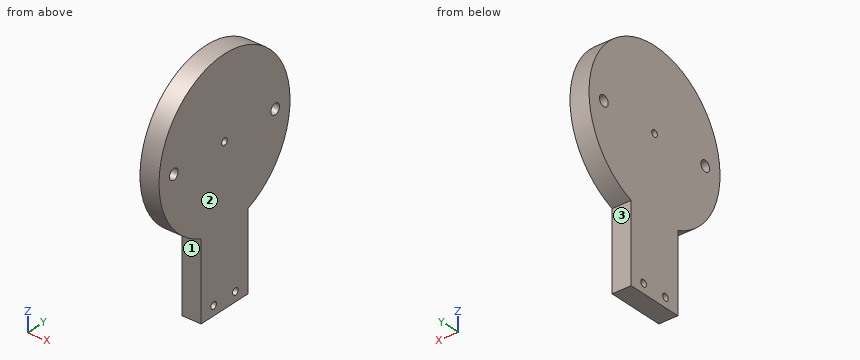
```python
from build123d import *

# Parameters (mm, degrees)
EXTRUDE_1_DEPTH     = 5
SKETCH_8_R          = 0.9
SKETCH_8_R_2        = 1.4
CUT_EXTRUDE_3_DEPTH = 10


with BuildPart() as part:
    # 스케치1 → 보스-돌출1 (new body)
    with BuildSketch(Plane(origin=(-9, 0, 0), x_dir=(0, -1, 0), z_dir=(-1, 0, 0))):
        with BuildLine():
            Line((-21, -18.122865071), (-21, 2.262089683))
            ThreePointArc((-21, 2.262089683), (-13.5, 42.877134929), (-6, 2.262089683))
            Line((-6, 2.262089683), (-6, -18.122865071))
            Line((-6, -18.122865071), (-21, -18.122865071))
        make_face()
    extrude(amount=-EXTRUDE_1_DEPTH)

    # 스케치8 → 컷-돌출3 (cut)
    with BuildSketch(Plane.ZY.offset(9)):
        with Locations((21.877134929, 13.5)):
            Circle(SKETCH_8_R)
        with Locations((-15.622865071, 17)):
            Circle(SKETCH_8_R)
        with Locations((-15.622865071, 10)):
            Circle(SKETCH_8_R)
        with Locations((21.877134929, 29.75)):
            Circle(SKETCH_8_R_2)
        with Locations((21.877134929, -2.75)):
            Circle(SKETCH_8_R_2)
    extrude(amount=-CUT_EXTRUDE_3_DEPTH, mode=Mode.SUBTRACT)


solid = part.part
```
Part model, mm, in its own coordinate system. Face numbers are marked on the shaded views. A direction names the side the tool comes from. Round coordinates to 2 decimals unless told otherwise and drop trailing zeros. Order: outer loops, then holes, each group sorted by start corner. A loop starts at its lowest first (then second) coordinate and runs counter-clockwise, first axis right, second up. Notation, with made-up numbers: M -27,15.5 L 29,15.5 A15 ccw 29,34.5 Z; hole C 6,-5 d10. An arc over 180 degrees is marked long. Answer in a Markdown table with one row per item. Add a question column.
Q1. Cut at B-B on x = -5.65. Give the cut face in (y, z), and give its area (3 significant figures).
Q2. Wall check: L1, parallel to Y at x = -7, z = -2; L2, parallel to Z at x = -7.45, y = 31; L3, parallel to Z at x = -6.6, y = 8. Give the ranges that are in metal, low to high. Write a range as from..to.
Q3. Cut at A-A on y = 30.5. Give the cut face in (x, z), and give its area (3 significant figures).
Q4. Pin check, flat tips, straight feed: pin 1 (1 mm diameter, centred on x = -5.5, y = 20, fed in from +Z); pin 2 (3 mm diameter, centred on x = -6.5, y = 8, fed in from +Z); pin 3 (1.1 mm diameter, centred on y = 17, z = -15.62, fed in from +X); pin 4 (3 mm diameter, centred on x = -7, z = 12.5, fed in from +Y). Stop position of each tip, or through.
Q5. Cut at C-C on z = -14. Give the cut face in (x, y), and give its area (3 significant figures).
Q6. 3-axis set-ups, long thin cutter, end or side, ignore diameter. For the marked faces 1, 2 and 3: which of +Z, -Z, +X, -X, +Y, -Y reach the whole face in a straight line?
Q7. Cut at D-D on y = 17. Give the cut face in (x, z), and give its area (3 significant figures).
Established:
| question | item | result |
|---|---|---|
| 1 | outline | M 6,-18.12 L 21,-18.12 L 21,2.26 A21 ccw long 6,2.26 Z; hole C -2.75,21.88 d2.8; hole C 10,-15.62 d1.8; hole C 13.5,21.88 d1.8; hole C 17,-15.62 d1.8; hole C 29.75,21.88 d2.8 |
| 1 | area | 1,660 mm2 |
| 2 | L1 | y = 6..21 |
| 2 | L2 | z = 10.27..21.25, 22.51..33.49 |
| 2 | L3 | z = -18.12..42.14 |
| 3 | outline | M -9,9.55 L -4,9.55 L -4,20.69 L -9,20.69 Z; M -9,23.06 L -4,23.06 L -4,34.21 L -9,34.21 Z |
| 3 | area | 111 mm2 |
| 4 | pin 1 | stops at z = 42 |
| 4 | pin 2 | stops at z = 42.49 |
| 4 | pin 3 | passes through |
| 4 | pin 4 | stops at y = 32.97 |
| 5 | outline | M -9,6 L -4,6 L -4,21 L -9,21 Z |
| 5 | area | 75.0 mm2 |
| 6 | face 1 | -Z, +X, -X, -Y |
| 6 | face 2 | +Z, -Z, +X, +Y, -Y |
| 6 | face 3 | -Z, +X, -X, +Y |
| 7 | outline | M -9,-18.12 L -4,-18.12 L -4,-16.52 L -9,-16.52 Z; M -9,-14.72 L -4,-14.72 L -4,42.58 L -9,42.58 Z |
| 7 | area | 295 mm2 |
